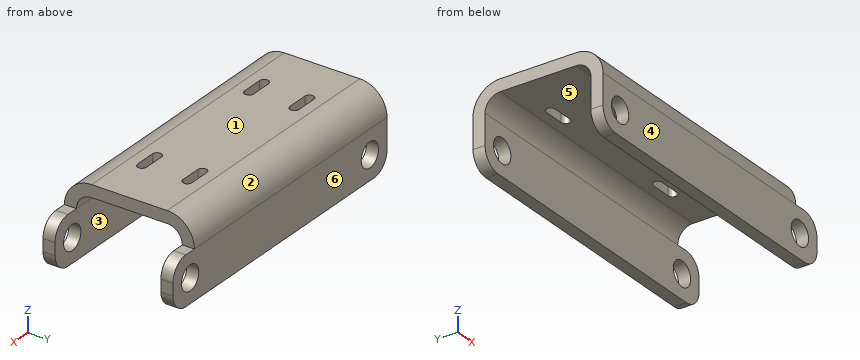
from build123d import *

# Parameters (mm, degrees)
SM_BASE_FLANGE_1_DEPTH = 100
SKETCH_4_R             = 4.05
CUT_EXTRUDE_1_DEPTH    = 112.687062814
SKETCH_5_W             = 10
SKETCH_5_H             = 9
CUT_EXTRUDE_2_DEPTH    = 112.687062814
FILLET_1_R             = 6
CUT_EXTRUDE_3_DEPTH    = 4


# Sheet-metal steps are written as plain solids
with BuildPart() as part:
    # Sketch 1 → Базовая кромка1 (new body)
    with BuildSketch(Plane(origin=(0, 0, 0), x_dir=(0, 0, -1), z_dir=(1, 0, 0))):
        with BuildLine():
            Line((25, -43), (9, -43))
            ThreePointArc((9, -43), (2.636038969, -40.363961031), (0, -34))
            Line((0, -34), (0, -9))
            ThreePointArc((0, -9), (2.636038969, -2.636038969), (9, 0))
            Line((9, 0), (25, 0))
            Line((25, 0), (25, -4))
            Line((25, -4), (9, -4))
            ThreePointArc((9, -4), (5.464466094, -5.464466094), (4, -9))
            Line((4, -9), (4, -34))
            ThreePointArc((4, -34), (5.464466094, -37.535533906), (9, -39))
            Line((9, -39), (25, -39))
            Line((25, -39), (25, -43))
        make_face()
    extrude(amount=SM_BASE_FLANGE_1_DEPTH)

    # Эскиз4 → Вырез-Вытянуть1 (cut, through all)
    with BuildSketch(Plane(origin=(0, 0, 0), x_dir=(1, 0, 0), z_dir=(0, 1, 0))):
        with Locations(Location((8, 17, 0), (0, 0, 270))):
            Circle(SKETCH_4_R)
        with Locations(Location((92, 17, 0), (0, 0, 270))):
            Circle(SKETCH_4_R)
    extrude(amount=-CUT_EXTRUDE_1_DEPTH, mode=Mode.SUBTRACT)

    # Эскиз5 → Вырез-Вытянуть2 (cut, through all)
    with BuildSketch(Plane.XZ.offset(43)):
        with Locations((95, -4.5)):
            Rectangle(SKETCH_5_W, SKETCH_5_H)
    extrude(amount=-CUT_EXTRUDE_2_DEPTH, mode=Mode.SUBTRACT)

    # Скругление1
    fillet_1_edges = [part.edges().sort_by_distance(p)[0] for p in [
        (0, -41, -25),
        (0, -2, -25),
        (100, -41, -25),
        (100, -2, -9),
        (100, -41, -9),
        (100, -2, -25),
    ]]
    fillet(fillet_1_edges, radius=FILLET_1_R)

    # Эскиз6 → Вырез-Вытянуть3 (cut)
    with BuildSketch(Plane.XY):
        with BuildLine():
            Line((16.5, -12.5), (23.5, -12.5))
            ThreePointArc((23.5, -12.5), (25, -14), (23.5, -15.5))
            Line((23.5, -15.5), (16.5, -15.5))
            ThreePointArc((16.5, -15.5), (15, -14), (16.5, -12.5))
        make_face()
        with BuildLine():
            Line((73.5, -12.5), (66.5, -12.5))
            ThreePointArc((66.5, -12.5), (65, -14), (66.5, -15.5))
            Line((66.5, -15.5), (73.5, -15.5))
            ThreePointArc((73.5, -15.5), (75, -14), (73.5, -12.5))
        make_face()
        with BuildLine():
            Line((73.5, -30.5), (66.5, -30.5))
            ThreePointArc((66.5, -30.5), (65, -29), (66.5, -27.5))
            Line((66.5, -27.5), (73.5, -27.5))
            ThreePointArc((73.5, -27.5), (75, -29), (73.5, -30.5))
        make_face()
        with BuildLine():
            Line((16.5, -30.5), (23.5, -30.5))
            ThreePointArc((23.5, -30.5), (25, -29), (23.5, -27.5))
            Line((23.5, -27.5), (16.5, -27.5))
            ThreePointArc((16.5, -27.5), (15, -29), (16.5, -30.5))
        make_face()
    extrude(amount=-CUT_EXTRUDE_3_DEPTH, mode=Mode.SUBTRACT)


solid = part.part
The listing builds one solid part. Answer for the finished solid, in the listing's coordinates (mm). Face numbers are marked on the shaded views. A direction names the side the tool comes from. Round coordinates to 2 decimals unless told otherwise and drop trailing zeros. Order: outer loops, then holes, each group sorted by start corner. A loop starts at its lowest first (then second) coordinate and runs counter-clockwise, first axis right, second up. Notation, with made-up numbers: (1.5, -6.75) -> (53.5, -6.75) arc R29 ccw to (53.5, 19.25) -> close; hole circle Ø11 at (65.25, 77). An arc over 180 degrees is marked (long way). Put each result on its own line as item: value.
Q1. Section D-D, the plane z = -17 is taken. Write down the section's boundary in (x, y).
Results list:
outline: (0, -43) -> (3.95, -43) -> (3.95, -39) -> (0, -39) -> close; (0, -4) -> (3.95, -4) -> (3.95, 0) -> (0, 0) -> close; (12.05, -43) -> (87.95, -43) -> (87.95, -39) -> (12.05, -39) -> close; (12.05, -4) -> (87.95, -4) -> (87.95, 0) -> (12.05, 0) -> close; (96.05, -43) -> (100, -43) -> (100, -39) -> (96.05, -39) -> close; (96.05, -4) -> (100, -4) -> (100, 0) -> (96.05, 0) -> close
Q2. Section B-B, the plane y = -29 is taken. Write down the section's boundary in (x, z).
Results list:
outline: (0, -4) -> (15, -4) -> (15, 0) -> (0, 0) -> close; (25, -4) -> (65, -4) -> (65, 0) -> (25, 0) -> close; (75, -4) -> (90, -4) -> (90, 0) -> (75, 0) -> close
Q3. Consider line 1 along X through (y, z) = (-2.65, -17); line 2 along Y through (x, z) = (21, -9.5); line 3 along X through (y, z) = (-41, -6.75). Determine where each line is inside the solid, lowest interval first.
Results list:
line 1: 0 to 3.95, 12.05 to 87.95, 96.05 to 100
line 2: -43 to -39, -4 to 0
line 3: 0 to 90
Q4. Which of the six approach directions +Z, -Z, +X, -X, +Y, -Y give full straight-line access (tool end or side, diameter ignored) to the marked faces 5 and 6?
Results list:
face 5: -Z, +X, -X
face 6: +Z, -Z, +X, -X, +Y
Q5. Section A-A, the plane x = 8 is taken. Write down the section's boundary in (y, z).
Results list:
outline: (-43, -25) -> (-39, -25) -> (-39, -21.05) -> (-43, -21.05) -> close; (-43, -12.95) -> (-39, -12.95) -> (-39, -9) arc R5 cw to (-34, -4) -> (-9, -4) arc R5 cw to (-4, -9) -> (-4, -12.95) -> (0, -12.95) -> (0, -9) arc R9 ccw to (-9, 0) -> (-34, 0) arc R9 ccw to (-43, -9) -> close; (-4, -25) -> (0, -25) -> (0, -21.05) -> (-4, -21.05) -> close
Q6. Determine the mould class of the marked faces 1, 2, 3 and 4 for opening direction Y: pulls with the +Y half, pulls with the -Y half, needs draft (parallel to the pull), parting line crosses it, or undercut.
Results list:
face 1: needs draft
face 2: pulls with the +Y half
face 3: undercut
face 4: pulls with the -Y half
Q7. Each of these flat-tipped pins is pushed along its axis until it touches: P1, Ø4.5, axis at x = 71, z = -2, coming from the +Y side; P2, Ø2, axis at x = 91.5, y = -41.5, coming from the +Z side; P3, Ø4.5, axis at x = 70.5, z = -3, coming from the -Y side; P4, Ø5, axis at x = 92, z = -17, coming from the +Y side. Where does it stop, or does it pass through?
Results list:
P1: y = -1.36
P2: z = -9
P3: y = -42.18
P4: through
Q8. Section C-C, the plane x = 92 is taken. Write down the section's boundary in (y, z).
Results list:
outline: (-43, -25) -> (-39, -25) -> (-39, -21.05) -> (-43, -21.05) -> close; (-43, -12.95) -> (-39, -12.95) -> (-39, -9) -> (-43, -9) -> close; (-4, -25) -> (0, -25) -> (0, -21.05) -> (-4, -21.05) -> close; (-4, -12.95) -> (0, -12.95) -> (0, -9) -> (-4, -9) -> close
